Can you work these out from the model? Positions are in its coordinate system, mm. A direction names the side the tool comes from. Round coordinates to 2 decimals unless told otherwise and drop trailing zeros. Order: outer loops, then holes, each group sorted by start corner. A loop starts at its lowest first (then second) coordinate and runs counter-clockwise, first axis right, second up. Notation, with made-up numbers: (-14.5, 9.5) - (15.5, 9.5) arc R28 ccw to (15.5, 43.5) - close; hole circle Ø2 at (81, -13.5). An arc over 180 degrees is marked (long way). Write item = value, one per line.
from build123d import *

# Parameters (mm, degrees)
F0_W     = 12.7
F0_H     = 12.7
F1_DEPTH = 190.5
F2_W     = 50.8
F2_H     = 50.8
F3_DEPTH = 12.7
F4_R     = 19.05
F5_DEPTH = 12.701
F6_R     = 19.04999
F7_R     = 3.175
F8_DEPTH = 31.751


# Not quite as in the source:
# - a fillet or chamfer is up to 0.001 mm smaller than in the source, because OpenCascade refuses the exact size


with BuildPart() as f1:
    # F0 (on Front) → F1 (new body)
    with BuildSketch(Plane.XZ):
        with Locations((6.35, -6.35)):
            Rectangle(F0_W, F0_H)
    extrude(amount=F1_DEPTH)

    # F2 (on face) → F3 (join)
    with BuildSketch(Plane.XY):
        with Locations((6.35, -215.9)):
            Rectangle(F2_W, F2_H)
    extrude(amount=-F3_DEPTH)

    # F4 (on face) → F5 (cut, through all)
    with BuildSketch(Plane.XY):
        with Locations((6.35, -215.9)):
            Circle(F4_R)
    extrude(amount=-F5_DEPTH, mode=Mode.SUBTRACT)

    # F6 (radius 19.05 in the source; OpenCascade refuses exactly that, so slightly less here)
    f6_edges = [f1.edges().sort_by_distance(p)[0] for p in [
        (31.75, -241.3, -6.35),
        (31.75, -190.5, -6.35),
        (-19.05, -241.3, -6.35),
        (-19.05, -190.5, -6.35),
    ]]
    fillet(f6_edges, radius=F6_R)

    # F7 (on face) → F8 (cut, through all)
    with BuildSketch(Plane.YZ.offset(12.7)):
        with Locations((0, -6.35)):
            Circle(F7_R)
    extrude(amount=-F8_DEPTH, mode=Mode.SUBTRACT)


solid = f1.part
(1) If I drill on line 1 (X direction, y = -135.5, z = -2); line 2 (Y direction, x = -8.5, z = -8.5); line 3 (Y direction, x = 6.35, z = -8.5), over which ranges is the centre line in solid material (lowest first)? Write a range as from..to.
Computed:
line_1 = 0..12.7
line_2 = -239.3..-227.83, -203.97..-192.5
line_3 = -241.3..-234.95, -196.85..-2.34
(2) Thinking about a two-plate mould opening in X: for faces 1 (the face through (26.32, -196.23, -6.44)), 2 (the face through (-13.62, -196.23, -6.44)), 3 (the face through (-7.691, -203.025, -6.261)), 4 (the face through (6, -119, -12.7)), which applies, +X half, -X half, draft (parallel to the pull), parting line (faces both ways), or undercut?
Computed:
face_1 = +X half
face_2 = -X half
face_3 = undercut
face_4 = draft
(3) On a 3-axis mill with a long thin cutter (end or side, diameter ignored), from which of +Z, -Z, +X, -X, +Y, -Y can I reach the whole of each face in a straight line? I mean faces 5 (the face through (12.7, -94, -6)), 6 (the face through (6.439, -3.174, -6.28)), 7 (the face through (0, -94, -6)). Say none if no direction works.
Computed:
face_5 = +Z, -Z, +X, +Y
face_6 = +X, -X, +Y
face_7 = +Z, -Z, -X, +Y
(4) If we section it at C-C (y = -215.9): Write out the boundary of the cut face in (x, z), plus the area to 3 significant figures.
Computed:
outline = (-19.05, -12.7) - (-12.7, -12.7) - (-12.7, 0) - (-19.05, 0) - close; (25.4, -12.7) - (31.75, -12.7) - (31.75, 0) - (25.4, 0) - close
area = 161 mm^2
(5) If we section it at A-A (x = 6.35): Write out the boundary of the cut face in (y, z) (3 decimals), plus the area to 3 significant figures.
Computed:
outline = (-241.3, -12.7) - (-234.95, -12.7) - (-234.95, 0) - (-241.3, 0) - close; (-196.85, -12.7) - (0, -12.7) - (0, -9.525) arc R3.175 cw to (0, -3.175) - (0, 0) - (-196.85, 0) - close
area = 2,560 mm^2
(6) If we section it at D-D (x = -10): Write out the boundary of the cut face in (y, z), plus the area to 3 significant figures.
Computed:
outline = (-238.46, -12.7) - (-225.68, -12.7) - (-225.68, 0) - (-238.46, 0) - close; (-206.12, -12.7) - (-193.34, -12.7) - (-193.34, 0) - (-206.12, 0) - close
area = 325 mm^2
(7) Will these pins go through, and if not, where does the flat tip stop? P1, Ø6.5, axis at y = -124, z = -7, coming from the -X side; P2, Ø3, axis at x = -1.5, y = -201, coming from the +Z side; P3, Ø4, axis at y = -114, z = -9.5, coming from the +X side; P4, Ø5, axis at x = 22, z = -2, coming from the -Y side (3 decimals).
Computed:
P1 = 0
P2 = through
P3 = 12.7
P4 = -240.045
